Read the model definition and answer for the solid it produces. Units are mm, in the model's axes. A direction names the side the tool comes from. Coordinates: 2 decimals unless noted, no trailing zeros. Loops run counter-clockwise (first coordinate to the right, second up) from the corner with the lowest first, then second, coordinate; pieces in that order, holes last. Notation, with made-up numbers: M 52,89 L 94,89 A15 cw 94,107 Z; hole C 37,-16.75 d4. An arc over 180 degrees is marked long. One line per item, written item: value. Start each with the question number.
```python
from build123d import *

# Parameters (mm, degrees)
SKETCH1_R           = 3.175
SKETCH1_R_2         = 1.8161
SKETCH1_R_3         = 7
BOSS_EXTRUDE1_DEPTH = 12.7


with BuildPart() as part:
    # Sketch1 → Boss-Extrude1 (new body)
    with BuildSketch(Plane.XY):
        with BuildLine():
            Line((-34.05, 9.525), (-15, 9.525))
            ThreePointArc((-15, 9.525), (0, -5.475), (15, 9.525))
            Line((15, 9.525), (34.05, 9.525))
            Line((34.05, 9.525), (34.05, 22.225))
            Line((34.05, 22.225), (46.75, 22.225))
            Line((46.75, 22.225), (46.75, 34.925))
            Line((46.75, 34.925), (-46.75, 34.925))
            Line((-46.75, 34.925), (-46.75, 22.225))
            Line((-46.75, 22.225), (-34.05, 22.225))
            Line((-34.05, 22.225), (-34.05, 9.525))
        make_face()
        with Locations((-40.4, 28.575)):
            Circle(SKETCH1_R, mode=Mode.SUBTRACT)
        with Locations((40.4, 28.575)):
            Circle(SKETCH1_R, mode=Mode.SUBTRACT)
        with Locations((8.248891971, 14.2875)):
            Circle(SKETCH1_R_2, mode=Mode.SUBTRACT)
        with Locations((-8.248891971, 14.2875)):
            Circle(SKETCH1_R_2, mode=Mode.SUBTRACT)
        Circle(SKETCH1_R_2, mode=Mode.SUBTRACT)
        with Locations((0, 9.525)):
            Circle(SKETCH1_R_3, mode=Mode.SUBTRACT)
    extrude(amount=BOSS_EXTRUDE1_DEPTH)


solid = part.part
```
1) A tool of negligible diameter and unlimited length cuts with its end or side. For faces 1 (the face through (39.712, 25.476, 6.261)), 2 (the face through (24, 9.525, 6)), 3 (the face through (-34.05, 16, 6)), from which of +Z, -Z, +X, -X, +Y, -Y can it reach the whole face along a straight path? Write none if from no direction.
2) Section B-B (x = -40.4) is taken. Determine the outline of the cut face in (y, z) (3 decimals), then the cut area to 3 significant figures.
3) Consider line 1 along Y through (x, z) = (0, 7.25) (3 decimals); line 2 along Y through (x, z) = (40.4, 10) (3 decimals); line 3 along X through (y, z) = (30, 8.5). Determine where each line is inside the solid, lowest interval first.
4) Section A-A (x = 0) is taken. Determine the outline of the cut face in (y, z) (3 decimals).
5) Section D-D (z = 4.5) is taken. Count the separate pieces of the cut face and the enclosed holes in it, then the cut area to 3 significant figures.
6) For a pull along Y with two mould halves and no side action, classify faces 4 (the face through (-9.6, 15.5, 6.3)), 5 (the face through (1, 34.925, 6)), 6 (the face through (40, 22.225, 6)), 7 (the face through (34.05, 16, 6)) as released by +Y, released by -Y, zero draft, split by the parting line, or undercut.
7) Section C-C (y = 27.5) is taken. Determine the outline of the cut face in (x, z), then the cut area to 3 significant figures.
8) Flat-ended cylindrical pins translate along their axes: pin 1 (6.5 mm diameter, centred on y = 12.5, z = 5, fed in from +X); pin 2 (4 mm diameter, centred on x = -41, z = 6.5, fed in from -Y) (3 decimals); pin 3 (6 mm diameter, centred on x = -16.5, z = 11.5, fed in from -Y). Find the tip coordinate at first contact, or state that the pin passes through.
Results found:
1. face 1: +Z, -Z
1. face 2: +Z, -Z, +X, -Y
1. face 3: +Z, -Z, -X, -Y
2. outline: M 22.225,0 L 25.4,0 L 25.4,12.7 L 22.225,12.7 Z; M 31.75,0 L 34.925,0 L 34.925,12.7 L 31.75,12.7 Z
2. area: 80.6 mm²
3. line 1: y = -5.475 to -1.816, 1.816 to 2.525, 16.525 to 34.925
3. line 2: y = 22.225 to 25.4, 31.75 to 34.925
3. line 3: x = -46.75 to -43.24, -37.56 to 37.56, 43.24 to 46.75
4. outline: M -5.475,0 L -1.816,0 L -1.816,12.7 L -5.475,12.7 Z; M 1.816,0 L 2.525,0 L 2.525,12.7 L 1.816,12.7 Z; M 16.525,0 L 34.925,0 L 34.925,12.7 L 16.525,12.7 Z
5. separate pieces: 1
5. enclosed holes: 6
5. area: 2,160 mm²
6. face 4: undercut
6. face 5: released by +Y
6. face 6: released by -Y
6. face 7: zero draft
7. outline: M -46.75,0 L -43.39,0 L -43.39,12.7 L -46.75,12.7 Z; M -37.41,0 L 37.41,0 L 37.41,12.7 L -37.41,12.7 Z; M 43.39,0 L 46.75,0 L 46.75,12.7 L 43.39,12.7 Z
7. area: 1,040 mm²
8. pin 1: stops at x = 34.05
8. pin 2: stops at y = 22.225
8. pin 3: stops at y = 2.99
